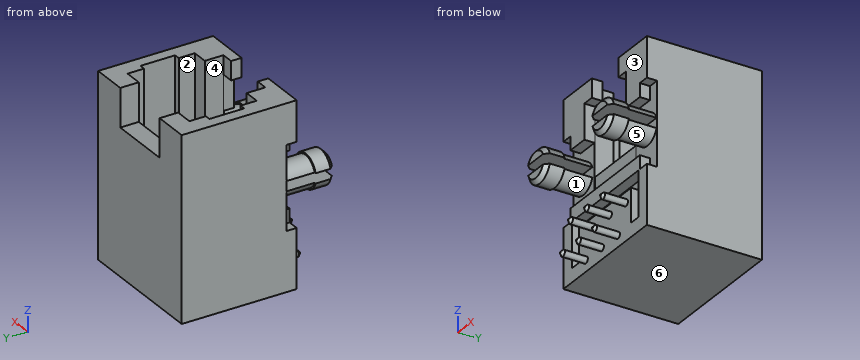
Autodesk Inventor part; units mm, degrees
ref_plane "Work Plane1" through (5.08, 0, 0) normal (1, 0, 0) x (0, 1, 0)
ref_plane "Work Plane2" through (-5.08, 0, 0) normal (1, 0, 0) x (0, 1, 0)
ref_plane "XZ Plane" through (0, 0, 0) normal (0, 1, 0) x (-1, 0, 0)
sketch "Sketch1" plane through (0, 0, 0) normal (0, 0, 1) x (1, 0, 0)
  line L0 (6.604, -5.715) -> (-6.604, -5.715)
  line L1 (-6.604, -5.715) -> (-6.604, 5.715)
  line L2 (-6.604, 5.715) -> (6.604, 5.715)
  line L3 (6.604, 5.715) -> (6.604, -5.715)
  line L4 (6.604, -5.715) -> (-6.604, 5.715) construction
  line L5 (-6.604, -5.715) -> (6.604, 5.715) construction
  point P0 (0, 0)
  dimension "d0" = 13.208
  dimension "d1" = 11.43
extrude "Extrusion1" add sketch "Sketch1" along normal mid plane 18.161
sketch "Sketch2" plane through (0, 0, 9.0805) normal (0, 0, 1) x (1, 0, 0)
  line L0 (0, -4.6736) -> (-3.3147, -4.6736)
  line L1 (-3.3147, -4.6736) -> (-3.3147, -2.8194)
  line L2 (-3.3147, -2.8194) -> (-4.8895, -2.8194)
  line L3 (-4.8895, -2.8194) -> (-4.8895, -1.2192)
  line L4 (-4.8895, -1.2192) -> (-5.461, -1.2192)
  line L5 (-5.461, -1.2192) -> (-5.461, 2.2352)
  line L6 (-5.461, 2.2352) -> (-4.8895, 2.2352)
  line L7 (-4.8895, 2.2352) -> (-4.8895, 3.8735)
  line L8 (-4.8895, 3.8735) -> (0, 3.8735)
  line L9 (0, 3.8735) -> (0, -4.6736) construction
  line L10 (6.604, 5.715) -> (-6.604, 5.715) construction
  line L11 (-6.604, -5.715) -> (6.604, -5.715) construction
  line L12 (0, -4.6736) -> (3.3147, -4.6736)
  line L13 (3.3147, -4.6736) -> (3.3147, -2.8194)
  line L14 (3.3147, -2.8194) -> (4.8895, -2.8194)
  line L15 (4.8895, -2.8194) -> (4.8895, -1.2192)
  line L16 (4.8895, -1.2192) -> (5.461, -1.2192)
  line L17 (5.461, -1.2192) -> (5.461, 2.2352)
  line L18 (5.461, 2.2352) -> (4.8895, 2.2352)
  line L19 (4.8895, 2.2352) -> (4.8895, 3.8735)
  line L20 (4.8895, 3.8735) -> (0, 3.8735)
  point P0 (0, 0)
  dimension "d17" = 1.8415
  dimension "d18" = 4.8895
  dimension "d19" = 5.461
  dimension "d20" = 1.0414
  dimension "d21" = 1.8542
  dimension "d22" = 4.4958
  dimension "d23" = 3.4798
  dimension "d24" = 3.3147
extrude "Extrusion2" cut sketch "Sketch2" against normal blind 8.6614
sketch "Sketch3" plane through (-6.604, 5.715, 9.0805) normal (0, 1, 0) x (1, 0, 0)
  line L0 (3.4925, 0) -> (9.7155, 0)
  line L1 (9.7155, 0) -> (9.7155, 3.81)
  line L2 (9.7155, 3.81) -> (3.4925, 3.81)
  line L3 (3.4925, 3.81) -> (3.4925, 0)
  line L4 (13.208, 0) -> (0, 0)
  point P0 (6.604, 9.0805)
  point P1 (6.604, 3.81)
  dimension "d27" = 6.223
  dimension "d28" = 3.81
extrude "Extrusion3" cut sketch "Sketch3" against normal up to surface (1.8415 mm away)
sketch "Sketch4" plane through (-6.604, -5.715, 9.0805) normal (0, -1, 0) x (1, 0, 0)
  line L0 (9.9187, 0) -> (3.2893, 0)
  line L1 (4.4958, 0) -> (4.4958, -1.8669)
  line L2 (4.4958, -1.8669) -> (3.3147, -1.8669)
  line L3 (3.3147, -1.8669) -> (3.3147, -10.9347)
  line L4 (3.3147, -10.9347) -> (9.8933, -10.9347)
  line L5 (9.8933, -10.9347) -> (9.8933, -1.8669)
  line L6 (9.8933, -1.8669) -> (8.7122, -1.8669)
  line L7 (8.7122, -1.8669) -> (8.7122, 0)
  line L8 (8.7122, 0) -> (4.4958, 0)
  point P0 (6.604, -9.0805)
  point P1 (6.604, 0)
  point P2 (6.604, -10.9347)
  dimension "d31" = 1.8669
  dimension "d32" = 4.2164
  dimension "d33" = 9.0678
  dimension "d34" = 6.5786
extrude "Extrusion4" cut sketch "Sketch4" against normal up to surface (1.0414 mm away)
sketch "Sketch5" plane through (-6.604, -5.715, -9.0805) normal (0, -1, 0) x (1, 0, 0)
  line L0 (0, 18.161) -> (0, 0)
  line L1 (0, 14.1605) -> (1.1176, 14.1605)
  line L2 (1.1176, 14.1605) -> (1.1176, 12.8143)
  line L3 (1.1176, 12.8143) -> (3.3147, 12.8143)
  line L4 (3.3147, 12.8143) -> (3.3147, 7.2263)
  line L5 (3.3147, 7.2263) -> (1.1176, 7.2263)
  line L6 (1.1176, 7.2263) -> (1.1176, 5.8801)
  line L7 (1.1176, 5.8801) -> (0, 5.8801)
  line L8 (0, 5.8801) -> (0, 14.1605)
  line L9 (3.3147, 7.2263) -> (3.3147, 16.2941) construction
  line L10 (6.604, 9.0805) -> (6.604, 17.5857) construction
  line L11 (1.3335, 1.3716) -> (1.3335, 5.8674)
  line L12 (1.3335, 5.8674) -> (11.8745, 5.8674)
  line L13 (11.8745, 5.8674) -> (11.8745, 1.3716)
  line L14 (11.8745, 1.3716) -> (10.7315, 1.3716)
  line L15 (10.7315, 1.3716) -> (10.7315, 4.7244)
  line L16 (10.7315, 4.7244) -> (2.4765, 4.7244)
  line L17 (2.4765, 4.7244) -> (2.4765, 1.3716)
  line L18 (2.4765, 1.3716) -> (1.3335, 1.3716)
  line L19 (13.208, 0) -> (0, 0)
  line L20 (13.208, 14.1605) -> (12.0904, 14.1605)
  line L21 (12.0904, 14.1605) -> (12.0904, 12.8143)
  line L22 (12.0904, 12.8143) -> (9.8933, 12.8143)
  line L23 (9.8933, 12.8143) -> (9.8933, 7.2263)
  line L24 (9.8933, 7.2263) -> (12.0904, 7.2263)
  line L25 (12.0904, 7.2263) -> (12.0904, 5.8801)
  line L26 (12.0904, 5.8801) -> (13.208, 5.8801)
  line L27 (13.208, 5.8801) -> (13.208, 14.1605)
  point P0 (6.604, 5.8674)
  dimension "d38" = 5.588
  dimension "d39" = 1.1176
  dimension "d41" = 8.2804
  dimension "d42" = 1.143
  dimension "d43" = 4.4958
  dimension "d44" = 1.143
  dimension "d45" = 1.3716
  dimension "d46" = 10.541
extrude "Extrusion5" cut sketch "Sketch5" against normal blind 1.016
ref_plane "Work Plane1" through (5.08, 0, 0) normal (1, 0, 0) x (0, 1, 0)
ref_plane "Work Plane2" through (-5.08, 0, 0) normal (1, 0, 0) x (0, 1, 0)
sketch "Sketch6" plane through (5.08, 0, 0) normal (1, 0, 0) x (0, 1, 0)
  line L0 (-4.6736, 2.5781) -> (-7.5565, 2.5781)
  line L1 (-7.5565, 2.5781) -> (-7.5565, 2.7305)
  line L2 (-7.5565, 2.7305) -> (-9.0297, 2.7305)
  line L3 (-9.0297, 2.7305) -> (-9.4361, 2.3241)
  line L4 (-9.4361, 2.3241) -> (-9.4361, 1.0541)
  line L5 (-9.4361, 1.0541) -> (-4.6736, 1.0541)
  line L6 (-4.6736, 2.5781) -> (-4.6736, 1.0541)
  line L7 (-4.6736, 9.0805) -> (-4.6736, 0.4191) construction
  line L8 (-4.6736, 9.0805) -> (-5.715, 9.0805) construction
  point P0 (0, 0)
  point P1 (0, 0)
  dimension "d51" = 1.524
  dimension "d53" = 1.6764
  dimension "d54" = 45
  dimension "d55" = 1.27
  dimension "d58" = 4.7625
  dimension "d59" = 1.4732
  dimension "d60" = 6.5024
revolve "Revolution1" add sketch "Sketch6" angle 360 about axis through (5.08, -9.4361, 1.0541) along (0, 1, 0)
sketch "Sketch7" plane through (-5.08, 0, 0) normal (1, 0, 0) x (0, 1, 0)
  line L0 (-4.6736, 2.5781) -> (-7.5565, 2.5781)
  line L1 (-7.5565, 2.5781) -> (-7.5565, 2.7305)
  line L2 (-7.5565, 2.7305) -> (-9.0297, 2.7305)
  line L3 (-9.0297, 2.7305) -> (-9.4361, 2.3241)
  line L4 (-9.4361, 2.3241) -> (-9.4361, 1.0541)
  line L5 (-9.4361, 1.0541) -> (-4.6736, 1.0541)
  line L6 (-4.6736, 2.5781) -> (-4.6736, 1.0541)
  line L7 (-4.6736, 9.0805) -> (-4.6736, 0.4191) construction
  line L8 (-4.6736, 9.0805) -> (-5.715, 9.0805) construction
  point P0 (0, 0)
  point P1 (0, 0)
  point P2 (0, 0)
  dimension "d62" = 1.524
  dimension "d63" = 1.6764
  dimension "d64" = 45
  dimension "d65" = 1.27
  dimension "d66" = 4.7625
  dimension "d67" = 1.4732
  dimension "d68" = 6.5024
revolve "Revolution2" add sketch "Sketch7" angle 360 about axis through (-5.08, -9.4361, 1.0541) along (0, 1, 0)
sketch "Sketch8" plane through (-5.08, -9.4361, 1.0541) normal (0, -1, 0) x (1, 0, 0)
  line L0 (-1.6764, 0.4953) -> (11.8364, 0.4953)
  line L1 (11.8364, 0.4953) -> (11.8364, -0.4953)
  line L2 (11.8364, -0.4953) -> (-1.6764, -0.4953)
  line L3 (-1.6764, -0.4953) -> (-1.6764, 0.4953)
  circle A0 centre (0, 0) radius 1.6764 construction
  circle A1 centre (10.16, 0) radius 1.6764 construction
  point P0 (5.08, -1.0541)
  point P1 (-1.6764, 0)
  point P2 (11.8364, 0)
  dimension "d70" = 0.9906
extrude "Extrusion6" cut sketch "Sketch8" against normal up to surface (4.7371 mm away)
sketch "Sketch9" plane through (-6.604, -5.715, -9.0805) normal (0, -1, 0) x (1, 0, 0)
  line L0 (9.7155, 14.351) -> (3.4925, 14.351)
  line L1 (9.7155, 18.161) -> (9.7155, 14.351)
  line L2 (3.4925, 14.351) -> (3.4925, 18.161)
  circle A0 centre (9.906, 3.6576) radius 0.3175
  circle A1 centre (8.636, 1.1176) radius 0.3175
  line L3 (9.7155, 14.351) -> (3.4925, 14.351)
  line L4 (13.208, 0) -> (13.208, 5.8801)
  line L5 (13.208, 0) -> (0, 0)
  circle A2 centre (7.366, 3.6576) radius 0.3175
  circle A3 centre (6.096, 1.1176) radius 0.3175
  circle A4 centre (4.826, 3.6576) radius 0.3175
  circle A5 centre (3.556, 1.1176) radius 0.3175
  point P0 (6.604, 9.0805)
  dimension "d73" = 3.302
  dimension "d74" = 2.54
  dimension "d75" = 1.27
  dimension "d76" = 3.6576
  dimension "d77" = 0.635
  dimension "d80" = 2.54
extrude "Extrusion7" add sketch "Sketch9" along normal blind 2.54 and the other way blind 1.27
chamfer "Chamfer1" distance 0.254 angle 45 6 edges at (1.7145, -8.255, -7.9629) (2.9845, -8.255, -5.4229) (0.4445, -8.255, -5.4229) (-0.8255, -8.255, -7.9629) (-2.0955, -8.255, -5.4229) (-3.3655, -8.255, -7.9629)
equation "\"d44\" = d42"
equation "\"d50\" = -d49"
properties part number "RJ12 - 90deg" material "Thermoplastic Resin"
Read the model definition and answer for the solid it produces. Units are mm, in the model's axes. Face numbers are marked on the shaded views. A direction names the side the tool comes from. Round coordinates to 2 decimals unless told otherwise and drop trailing zeros. Loops run counter-clockwise (first coordinate to the right, second up) from the corner with the lowest first, then second, coordinate; pieces in that order, holes last.
Q1. Each of these flat-tipped pins is pushed along its axis until it touches: pin 1 (1 mm diameter, centred on x = 4.5, y = -7, fed in from +Z); pin 2 (1 mm diameter, centred on x = 5, y = -8, fed in from -Z); pin 3 (0.5 mm diameter, centred on y = -5, z = 4.5, fed in from +X). Where does it stop, or does it pass through?
Q2. Consider probe 1 along X at (y, z) = (0, 3); probe 2 along X at (y, z) = (-1.75, 6.25); probe 3 along Y at (x, z) = (4.5, 7.5) (1 decimal). Determine where each line is inside the solid, lowest interval first.
Q3. Which of the six approach directions +Z, -Z, +X, -X, +Y, -Y give full straight-line access (tool end or side, diameter ignored) to the marked faces 1, 2 and 3?
Q4. Section B-B on y = -8.5 is taken. Write down the section's boundary in (x, z), and give its area (3 significant figures).
Q5. Determine the mould class of the marked faces 4, 5 and 6 for opening direction Z: released by +Z, released by -Z, zero draft, split by the parting line, or undercut.
Q6. Section C-C on y = 2.75 is taken. Write down the section's boundary in (x, z), and give its area (3 significant figures).
Output:
1. pin 1: stops at z = 2.58
1. pin 2: stops at z = -0.62
1. pin 3: stops at x = 5.49
2. probe 1: x = -6.6 to -5.46, 5.46 to 6.6
2. probe 2: x = -6.6 to -4.89, 4.89 to 6.6
2. probe 3: y = -5.7 to -2.8, 3.9 to 5.7
3. face 1: none
3. face 2: +Z
3. face 3: +Z, +X, -X, -Y
4. outline: (-6.68, 0.56) arc R1.68 ccw to (-3.48, 0.56) - close; (-6.68, 1.55) - (-3.48, 1.55) arc R1.68 ccw to start; (3.48, 0.56) arc R1.68 ccw to (6.68, 0.56) - close; (3.48, 1.55) - (6.68, 1.55) arc R1.68 ccw to start
4. area: 11.1 mm2
5. face 4: zero draft
5. face 5: undercut
5. face 6: released by -Z
6. outline: (-6.6, -9.08) - (6.6, -9.08) - (6.6, 9.08) - (4.89, 9.08) - (4.89, 0.42) - (-4.89, 0.42) - (-4.89, 9.08) - (-6.6, 9.08) - close
6. area: 155 mm2
